Can you work these out from the model? Positions are in its coordinate system, mm. A direction names the side the tool comes from. Coordinates: 2 decimals unless noted, no trailing zeros. Write each loop counter-clockwise with the first axis right and the second up, starting at its lowest first coordinate (ties: lowest second). Pieces come first, ordered by that corner, then holes. Notation, with made-up numbers: (10, -25.75) -> (25, -25.75) arc R13 cw to (25, -16.75) -> close; hole circle Ø3 at (-2, 15). An arc over 180 degrees is marked (long way). Use one line per item in the form item = value.
Autodesk Inventor part; units mm, degrees
ref_plane "YZ Plane" through (0, 0, 0) normal (1, 0, 0) x (0, 1, 0)
ref_plane "XZ Plane" through (0, 0, 0) normal (0, 1, 0) x (-1, 0, 0)
ref_plane "XY Plane" through (0, 0, 0) normal (0, 0, 1) x (1, 0, 0)
sketch "Boceto1" plane through (0, 0, 0) normal (1, 0, 0) x (0, 1, 0)
  circle A0 centre (0, 0) radius 12.5
  circle A1 centre (0, 0) radius 6.75
  dimension "d0" = 25
  dimension "d1" = 13.5
extrude "Extrusión1" add sketch "Boceto1" against normal blind 90 contours A1
extrude "Extrusión2" add sketch "Boceto1" along normal mid plane 160
sketch "Boceto2" plane through (0, 0, 0) normal (1, 0, 0) x (0, 0, -1)
  circle A0 centre (0, 0) radius 6.75
  dimension "d6" = 13.5
extrude "Extrusión3" add sketch "Boceto2" along normal blind 100
properties part number "eje" material "Acero, no aleado"
Q1. If I drill on line 1 (X direction, y = -0.75, z = -7); line 2 (Z direction, x = 3, y = -0.5); line 3 (Y direction, x = -18.5, z = -10.25), over which ranges is the centre line in solid material (lowest first)? Write a range as from..to.
Return value:
line_1 = -80..80
line_2 = -12.49..12.49
line_3 = -7.15..7.15
Q2. Suppose I cut it at C-C (x = -71). Write out the boundary of the cut face in (y, z).
Return value:
outline = circle Ø25 at (0, 0)
Q3. For faces 1 (the flat face through (100, 0, 0)), 2 (the cylindrical face through (89.86, 6.59, 1.46)), 3 (the flat face through (-80, 5, -5)), which set-ups out of +Z, -Z, +X, -X, +Y, -Y let a thin tool reach every point of the face, with its end or its side?
Return value:
face_1 = +Z, -Z, +X, +Y, -Y
face_2 = +X
face_3 = -X
Q4. Will these pins go through, and if not, where does the flat tip stop? pin 1 (1 mm diameter, centred on x = -10.5, y = 1.5, fed in from -Z); pin 2 (8 mm diameter, centred on x = 68, y = -5.5, fed in from +Z); pin 3 (6 mm diameter, centred on x = -61, z = -7, fed in from +Y).
Return value:
pin_1 = -12.46
pin_2 = 12.41
pin_3 = 11.84
Q5. Suppose I cut it at A-A (y = 0). Write out the boundary of the cut face in (x, z).
Return value:
outline = (-90, -6.75) -> (-80, -6.75) -> (-80, -12.5) -> (80, -12.5) -> (80, -6.75) -> (100, -6.75) -> (100, 6.75) -> (80, 6.75) -> (80, 12.5) -> (-80, 12.5) -> (-80, 6.75) -> (-90, 6.75) -> close
Q6. Suppose I cut it at D-D (z = 10.25). Write out the boundary of the cut face in (x, y).
Return value:
outline = (-80, -7.15) -> (80, -7.15) -> (80, 7.15) -> (-80, 7.15) -> close
